Design review of the part built by this model. Coordinates are the model's own, in mm. A direction names the side the tool comes from. Give positions to 0.01 mm unless a question says otherwise; leave off trailing zeros. Order: outer loops, then holes, each group sorted by start corner. A loop starts at its lowest first (then second) coordinate and runs counter-clockwise, first axis right, second up. Notation, with made-up numbers: M 75,43.5 L 133,43.5 A26 cw 133,60.5 Z; hole C 25,13.5 d5. An arc over 180 degrees is marked long. Answer as a JSON object with one key per item and string values.
from build123d import *

# Parameters (mm, degrees)
PAD017_DEPTH           = 5
PAD020_DEPTH           = 6.25
SKETCH105_W            = 7.5
SKETCH105_H            = 1.65
PAD074_DEPTH           = 5
SKETCH102_W            = 7.5
SKETCH102_H            = 1.65
PAD075_DEPTH           = 2.1
SKETCH103_W            = 2.1
SKETCH103_H            = 1.65
PAD076_DEPTH           = 5
SKETCH104_W            = 7.5
SKETCH104_H            = 1.65
PAD077_DEPTH           = 5
LINEARPATTERN024_COUNT = 2
LINEARPATTERN024_PITCH = 3.3
CHAMFER014_SIZE        = 1


with BuildPart() as obj1:
    # Sketch034 → Pad017 (new body)
    with BuildSketch(Plane.XY):
        with BuildLine():
            Line((-1.35, -1.8), (-1.35, 6))
            ThreePointArc((0, 7.35), (-0.954594, 6.954594), (-1.35, 6))
            Line((0, 9), (0, 7.35))
            Line((-2.6, 9), (0, 9))
            Line((-2.6, -1.8), (-2.6, 9))
            Line((-3.85, -1.8), (-2.6, -1.8))
            ThreePointArc((-3.85, -1.8), (-3.439949, -2.789949), (-2.45, -3.2))
            Line((-1.35, -3.2), (-2.45, -3.2))
            Line((-1.35, -1.8), (-1.35, -3.2))
        make_face()
    extrude(amount=PAD017_DEPTH)

    # Sketch037 → Pad020 (join)
    with BuildSketch(Plane.XY):
        Polygon((-1.35, 0.2), (-1.35, 1.6), (-2.6, 1.6), (-3.85, 1.6), (-3, 0.2), (-2.6, 0.2), align=None)
    extrude(amount=PAD020_DEPTH)


with BuildPart() as obj2:
    # Mirror001: instance of _obj1
    add(obj1.part.mirror(Plane(origin=(0, 0, 0), x_dir=(0, 1, 0), z_dir=(-1, 0, 0))))


with BuildPart() as body039:
    # Fusion001 base: copy of _obj1
    add(obj1.part)

    # Fusion001: union _obj2)
    add(obj2.part)

    # Sketch105 → Pad074 (new body)
    with BuildSketch(Plane.XY):
        with Locations((1.15, 8.175)):
            Rectangle(SKETCH105_W, SKETCH105_H)
    extrude(amount=PAD074_DEPTH)

    # Sketch102 → Pad075 (join)
    with BuildSketch(Plane.XY):
        with Locations((1.15, 9.825)):
            Rectangle(SKETCH102_W, SKETCH102_H)
    pad075 = extrude(amount=PAD075_DEPTH)

    # Sketch103 → Pad076 (join)
    with BuildSketch(Plane.XY):
        with Locations((3.85, 9.825)):
            Rectangle(SKETCH103_W, SKETCH103_H)
    pad076 = extrude(amount=PAD076_DEPTH)

    # Sketch104 → Pad077 (join)
    with BuildSketch(Plane.XY):
        with Locations((1.15, 11.475)):
            Rectangle(SKETCH104_W, SKETCH104_H)
    pad077 = extrude(amount=PAD077_DEPTH)

    # LinearPattern024: Pad077, Pad076, Pad075 ×2
    with Locations(*[(0, i * LINEARPATTERN024_PITCH, 0) for i in range(1, LINEARPATTERN024_COUNT)]):
        add(pad077)
        add(pad076)
        add(pad075)

    # Chamfer014
    chamfer014_edges = [body039.edges().sort_by_distance(p)[0] for p in [
        (-2.6, 8.175, 5),
        (-2.6, 11.475, 5),
        (-2.6, 14.775, 5),
    ]]
    chamfer(chamfer014_edges, length=CHAMFER014_SIZE)


solid = body039.part
(1) Draft analysis for pull direction Y (two halves, no side actions). For faces 5 (the flat face through (4, 7.35, 2)), 6 (the cylindrical face through (-3.45, -2.78, 2.46)), 7 (the flat face through (0, 8, 0)), state which applies: +Y half, -Y half, draft (parallel to the pull), parting line (faces both ways), or undercut.
Checked values:
{"face 5": "undercut", "face 6": "-Y half", "face 7": "draft"}
(2) Tool access review of faces 1 (the flat face through (-2.1, 5.2, 4.5)), 2 (the flat face through (0, 10, 2.1)), 3 (the flat face through (2.6, -1, 2)), 4 (the flat face through (-2.6, 8.5, 2)): name each direction out of +Z, -Z, +X, -X, +Y, -Y from which nothing blocks a thin tool from reaching the whole face with its end or side.
Checked values:
{"face 1": "+Z, -X, +Y", "face 2": "+Z, -X", "face 3": "+Z, -Z, +X", "face 4": "+Z, -Z, -X, +Y"}
(3) We need section C-C (x = 1.75). Write out the cut boundary in (y, z).
Checked values:
{"outline": "M -3.2,0 L 15.6,0 L 15.6,5 L 13.95,5 L 13.95,2.1 L 12.3,2.1 L 12.3,5 L 10.65,5 L 10.65,2.1 L 9,2.1 L 9,5 L 1.6,5 L 1.6,6.25 L 0.2,6.25 L 0.2,5 L -3.2,5 Z"}
(4) Insertion check: pin 1 (1.8 mm diameter, centred on x = -0.5, y = 10, fed in from +Z); pin 2 (0.6 mm diameter, centred on y = -1, z = 2, fed in from +X); pin 3 (1.5 mm diameter, centred on x = 0, z = 1, fed in from -Y). Each pin has a flat end and moves straight along its axis. Give the tip position at first contact, or say it passes through.
Checked values:
{"pin 1": "stops at z = 5", "pin 2": "stops at x = 2.6", "pin 3": "stops at y = 7.12"}
(5) To check wall thickness, follow L1, parallel to Y at x = -1.5, z = 3; L2, parallel to X at y = 2.5, z = 2.75; L3, parallel to Y at x = 3.5, z = 2.25. State the ranges of each line that lie inside material, in increasing order. Write a range as from..to.
Checked values:
{"L1": "y = -3.2..9, 10.65..12.3, 13.95..15.6", "L2": "x = -2.6..-1.35, 1.35..2.6", "L3": "y = -2.73..-1.8, 1.02..1.6, 7.35..15.6"}
(6) We need section A-A (y = 2.5). Write out the cut boundary in (x, z).
Checked values:
{"outline": "M -2.6,0 L -1.35,0 L -1.35,5 L -1.6,5 L -2.6,4 Z; M 1.35,0 L 2.6,0 L 2.6,5 L 1.35,5 Z"}
(7) We need section D-D (y = 9.5). Write out the cut boundary in (x, z), plus the area to 3 significant figures.
Checked values:
{"outline": "M -2.6,0 L 4.9,0 L 4.9,5 L 2.8,5 L 2.8,2.1 L -2.6,2.1 Z", "area": "21.8 mm^2"}
